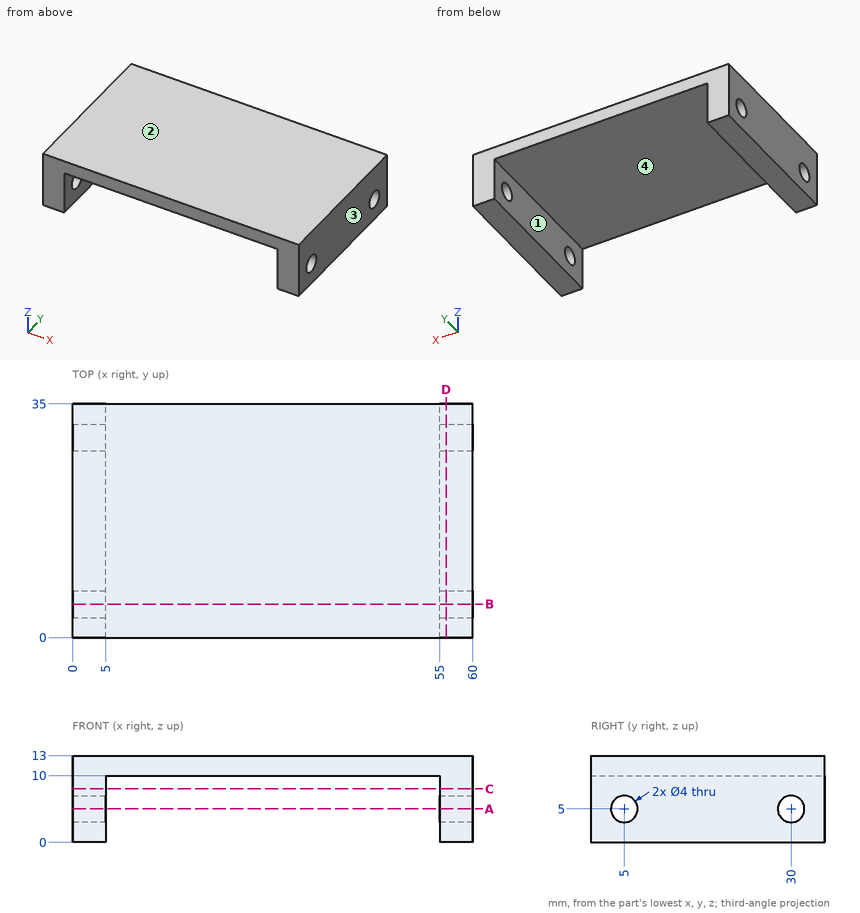
Input: dimensioned drawing with shaded views. Units: mm. Origin: part minimum x, y, z. Give positions to 0.01 mm unless a question says otherwise; leave off trailing zeros. Write each loop counter-clockwise with the first axis right and the second up, starting at its lowest first coordinate (ties: lowest second). Pieces come first, ordered by that corner, then holes. Notation, with made-up numbers: M -25.5,-32 L -3.5,-32 A35 cw -3.5,1 Z; hole C 29,35.25 d5. An arc over 180 degrees is marked long. Return JSON: item names as keys, results as strings. Group by question number.
1) Cut plane B-B, the plane y = 5. Output: boundary loops of the cut face in (x, z), plus the area to 3 significant figures.
2) Cut plane C-C, the plane z = 8. Output: boundary loops of the cut face in (x, y), plus the area to 3 significant figures.
3) Pin query (flat end, axial travel): P1, Ø1, axis at x = 32.5, y = 19, coming from the -Z side; P2, Ø3.5, axis at y = 5, z = 5, coming from the +X side. Return the tip coordinate at first contact, or that it passes through.
4) Pull-direction query (X, two-part tool) for the marked faces 1, 2, 3 and 4; classes: pulls with the +X half, pulls with the -X half, needs draft (parallel to the pull), parting line crosses it, or undercut.
5) Cut plane A-A, the plane z = 5. Output: boundary loops of the cut face in (x, y).
6) Material intervals for line 1 along Y through (x, z) = (3.65, 5); line 2 along X through (y, z) = (10, 5); line 3 along Z through (x, y) = (7.5, 13.5), sorted ascending. Write a range as [from, to].
7) Cut plane D-D, the plane x = 56. Output: boundary loops of the cut face in (y, z), plus the area to 3 significant figures.
Recorded:
{
 "1": {"outline": "M 0,0 L 5,0 L 5,3 L 0,3 Z; M 0,7 L 5,7 L 5,10 L 55,10 L 55,7 L 60,7 L 60,13 L 0,13 Z; M 55,0 L 60,0 L 60,3 L 55,3 Z", "area": "240 mm²"},
 "2": {"outline": "M 0,0 L 5,0 L 5,35 L 0,35 Z; M 55,0 L 60,0 L 60,35 L 55,35 Z", "area": "350 mm²"},
 "3": {"P1": "stops at z = 10", "P2": "passes through"},
 "4": {"face 1": "undercut", "face 2": "needs draft", "face 3": "pulls with the +X half", "face 4": "undercut"},
 "5": {"outline": "M 0,0 L 5,0 L 5,3 L 0,3 Z; M 0,7 L 5,7 L 5,28 L 0,28 Z; M 0,32 L 5,32 L 5,35 L 0,35 Z; M 55,0 L 60,0 L 60,3 L 55,3 Z; M 55,7 L 60,7 L 60,28 L 55,28 Z; M 55,32 L 60,32 L 60,35 L 55,35 Z"},
 "6": {"line 1": "y = [0, 3], [7, 28], [32, 35]", "line 2": "x = [0, 5], [55, 60]", "line 3": "z = [10, 13]"},
 "7": {"outline": "M 0,0 L 35,0 L 35,13 L 0,13 Z; hole C 5,5 d4; hole C 30,5 d4", "area": "430 mm²"}
}
